Check sheet for the modelled part. Datum: model origin and axes. Units: mm. Face numbers are marked on the shaded views. A direction names the side the tool comes from. Coordinates: 2 decimals unless noted, no trailing zeros. Loops run counter-clockwise (first coordinate to the right, second up) from the corner with the lowest first, then second, coordinate; pieces in that order, holes last. Notation, with made-up numbers: (60, 20) -> (95, 20) arc R26 cw to (95, 34) -> close; hole circle Ø1 at (-28, -19.5). An arc over 180 degrees is marked (long way). Use CSV: the item, a comma, the result in double quotes.
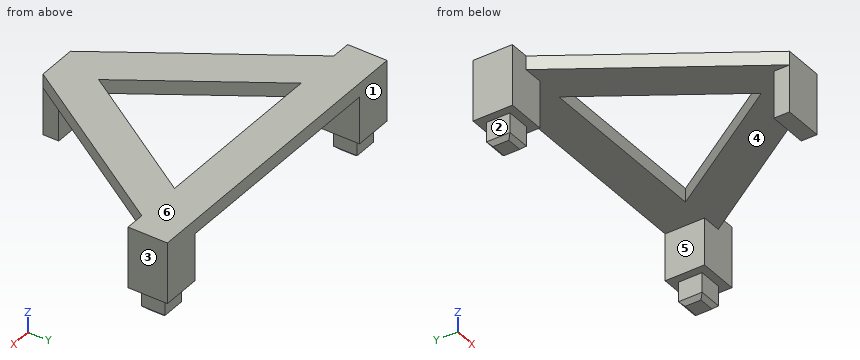
Autodesk Inventor part; units mm, degrees
ref_plane "YZ Plane" through (0, 0, 0) normal (1, 0, 0) x (0, 1, 0)
ref_plane "XZ Plane" through (0, 0, 0) normal (0, 1, 0) x (-1, 0, 0)
ref_plane "XY Plane" through (0, 0, 0) normal (0, 0, 1) x (1, 0, 0)
sketch "Sketch1" plane through (0, 0, 0) normal (0, 0, 1) x (1, 0, 0)
  line L0 (20.5636, -7.0902) -> (-9.4364, -7.0902)
  line L1 (-9.4364, -7.0902) -> (-9.4364, 33.4098)
  line L2 (-9.4364, 33.4098) -> (20.5636, 33.4098)
  line L3 (20.5636, 33.4098) -> (20.5636, -7.0902)
  line L4 (20.5636, 13.9098) -> (-9.4364, 13.9098)
  line L5 (20.5636, 13.9098) -> (25.5636, 13.9098)
  line L6 (25.5636, 13.9098) -> (25.5636, 18.9098)
  line L7 (25.5636, 18.9098) -> (20.5636, 18.9098)
  line L8 (5.5636, -7.0902) -> (5.5636, 33.4098)
  line L9 (-9.4364, 13.9098) -> (-14.4364, 13.9098)
  line L10 (-14.4364, 13.9098) -> (-14.4364, 18.9098)
  line L11 (-14.4364, 18.9098) -> (-9.4364, 18.9098)
  line L12 (3.0636, -7.0902) -> (3.0636, -9.0902)
  line L13 (3.0636, -9.0902) -> (8.0636, -9.0902)
  line L14 (8.0636, -9.0902) -> (8.0636, -7.0902)
  line L15 (3.0636, -9.0902) -> (-11.9364, 13.9098)
  line L16 (8.0636, -9.0902) -> (23.0636, 13.9098)
  line L17 (-9.4364, 18.9098) -> (20.5636, 18.9098)
  line L18 (17.0943, 13.9098) -> (5.5636, -3.7706)
  line L19 (5.5636, -3.7706) -> (-5.967, 13.9098)
  point P0 (0, 0)
  point P1 (20.5636, 9.5176)
  point P2 (-9.4364, 9.5176)
  point P3 (5.5636, -1.9167)
  point P4 (-9.4364, 13.9098)
  dimension "d0" = 30
  dimension "d1" = 40.5
  dimension "d4" = 5
  dimension "d5" = 5
  dimension "d7" = 2
  dimension "d8" = 5
  dimension "d9" = 2.5
  dimension "d12" = 23
  dimension "d15" = 5
extrude "Extrusion1" add sketch "Sketch1" along normal blind 1.75 contours L14 L13 L12 L0 | L0 L8 L18 L4 L3 L16 | L0 L16 L14 | L0 L15 L1 L4 L19 L8 | L12 L15 L0 | L3 L5 L16 | L8 L17 L3 L4 | L4 L1 L17 L8 | L3 L7 L6 L5 | L15 L9 L1 | L9 L10 L11 L1
extrude "Extrusion2" add sketch "Sketch1" against normal blind 6 contours L14 L13 L12 L0
extrude "Extrusion3" add sketch "Sketch1" against normal blind 6 contours L3 L7 L6 L5 | L9 L10 L11 L1
sketch "Sketch3" plane through (0, 0, -6) normal (0, 0, -1) x (-1, 0, 0)
  line L0 (9.4364, 13.9098) -> (14.4364, 13.9098)
  line L1 (9.4364, 13.9098) -> (14.4364, 13.9098)
  line L2 (14.4364, 13.9098) -> (14.4364, 18.9098)
  line L3 (14.4364, 18.9098) -> (9.4364, 18.9098)
  line L4 (9.4364, 18.9098) -> (9.4364, 13.9098)
  line L5 (-20.5636, 13.9098) -> (-23.0636, 13.9098)
  line L6 (-25.5636, 18.9098) -> (-25.5636, 13.9098)
  line L7 (-20.5636, 13.9098) -> (-25.5636, 13.9098)
  line L8 (-25.5636, 13.9098) -> (-25.5636, 18.9098)
  line L9 (-25.5636, 18.9098) -> (-20.5636, 18.9098)
  line L10 (-20.5636, 18.9098) -> (-20.5636, 13.9098)
  line L11 (-21.5636, 14.9098) -> (-24.5636, 14.9098)
  line L12 (-24.5636, 14.9098) -> (-24.5636, 17.9098)
  line L13 (-24.5636, 17.9098) -> (-21.5636, 17.9098)
  line L14 (-21.5636, 17.9098) -> (-21.5636, 14.9098)
  line L15 (13.4364, 17.9098) -> (13.4364, 14.9098)
  line L16 (13.4364, 14.9098) -> (10.4364, 14.9098)
  line L17 (10.4364, 14.9098) -> (10.4364, 17.9098)
  line L18 (10.4364, 17.9098) -> (13.4364, 17.9098)
  point P0 (0, 0)
  dimension "d23" = 1
  dimension "d24" = 1
extrude "Extrusion4" add sketch "Sketch3" along normal blind 3 contours L11 L12 L13 L14 | L15 L16 L17 L18
chamfer "Chamfer2" distance 0.5 angle 45 8 edges at (23.0636, 17.9098, -9) (24.5636, 16.4098, -9) (21.5636, 16.4098, -9) (23.0636, 14.9098, -9) (-13.4364, 16.4098, -9) (-11.9364, 17.9098, -9) (-10.4364, 16.4098, -9) (-11.9364, 14.9098, -9)
equation "\"d5\" = d4"
equation "\"d9\" = 0.5 * d8"
properties part number "BareCalibrationClipBatteryMount"
1) Thickness scan on line 1 along X through (y, z) = (16.5, -7.25); line 2 along X through (y, z) = (17, -2); line 3 along Y through (x, z) = (-12, -7.5). Record the ranges inside material, lowest first. Write a range as from..to.
Answer below:
line 1,"x = -13.44..-10.44, 21.56..24.56"
line 2,"x = -14.44..-9.44, 20.56..25.56"
line 3,"y = 14.91..17.91"
2) Cross-section at B-B on x = 6. Record the boundary of the cut face in (y, z), and give its area (3 significant figures).
Answer below:
outline,"(-9.09, -6) -> (-7.09, -6) -> (-7.09, 0) -> (-3.1, 0) -> (-3.1, 1.75) -> (-9.09, 1.75) -> close; (13.91, 0) -> (18.91, 0) -> (18.91, 1.75) -> (13.91, 1.75) -> close"
area,"31.2 mm²"
3) Access from +Z, -Z, +X, -X, +Y, -Y to the whole of each face (thin tool, end or side, straight path). Record for the marked faces 5 and 6.
Answer below:
face 5,"-Z, +Y, -Y"
face 6,"+Z, +X, -X, +Y, -Y"
4) Go/stop test with flat-tipped pins: pin 1 Ø3 at (x, z) = (22.5, -7) entering from +Y; pin 2 Ø2 at (x, y) = (6.5, -8) entering from -Z; pin 3 Ø1 at (x, y) = (14, -4.5) entering from -Z; pin 4 Ø14 at (x, y) = (13.5, 9) entering from -Z. Record where each tip stops, or that it passes through.
Answer below:
pin 1,"stops at y = 18.91"
pin 2,"stops at z = -6"
pin 3,"passes through"
pin 4,"stops at z = 0"
5) Cross-section at C-C on y = 3.5. Record the boundary of the cut face in (x, z).
Answer below:
outline,"(-5.15, 0) -> (0.82, 0) -> (0.82, 1.75) -> (-5.15, 1.75) -> close; (10.31, 0) -> (16.27, 0) -> (16.27, 1.75) -> (10.31, 1.75) -> close"
6) Cross-section at D-D on x = -10. Record the boundary of the cut face in (y, z), and give its area (3 significant figures).
Answer below:
outline,"(10.94, 0) -> (13.91, 0) -> (13.91, -6) -> (18.91, -6) -> (18.91, 1.75) -> (10.94, 1.75) -> close"
area,"43.9 mm²"
7) Draft check along X on the marked faces 1, 2, 3 and 4. Enter one of: released by +X, released by -X, zero draft, split by the parting line, or undercut.
Answer below:
face 1,"zero draft"
face 2,"released by -X"
face 3,"released by +X"
face 4,"undercut"
8) Cross-section at A-A on z = -1.75. Record the boundary of the cut face in (x, y), and give its area (3 significant figures).
Answer below:
outline,"(-14.44, 13.91) -> (-9.44, 13.91) -> (-9.44, 18.91) -> (-14.44, 18.91) -> close; (3.06, -9.09) -> (8.06, -9.09) -> (8.06, -7.09) -> (3.06, -7.09) -> close; (20.56, 13.91) -> (25.56, 13.91) -> (25.56, 18.91) -> (20.56, 18.91) -> close"
area,"60.0 mm²"
